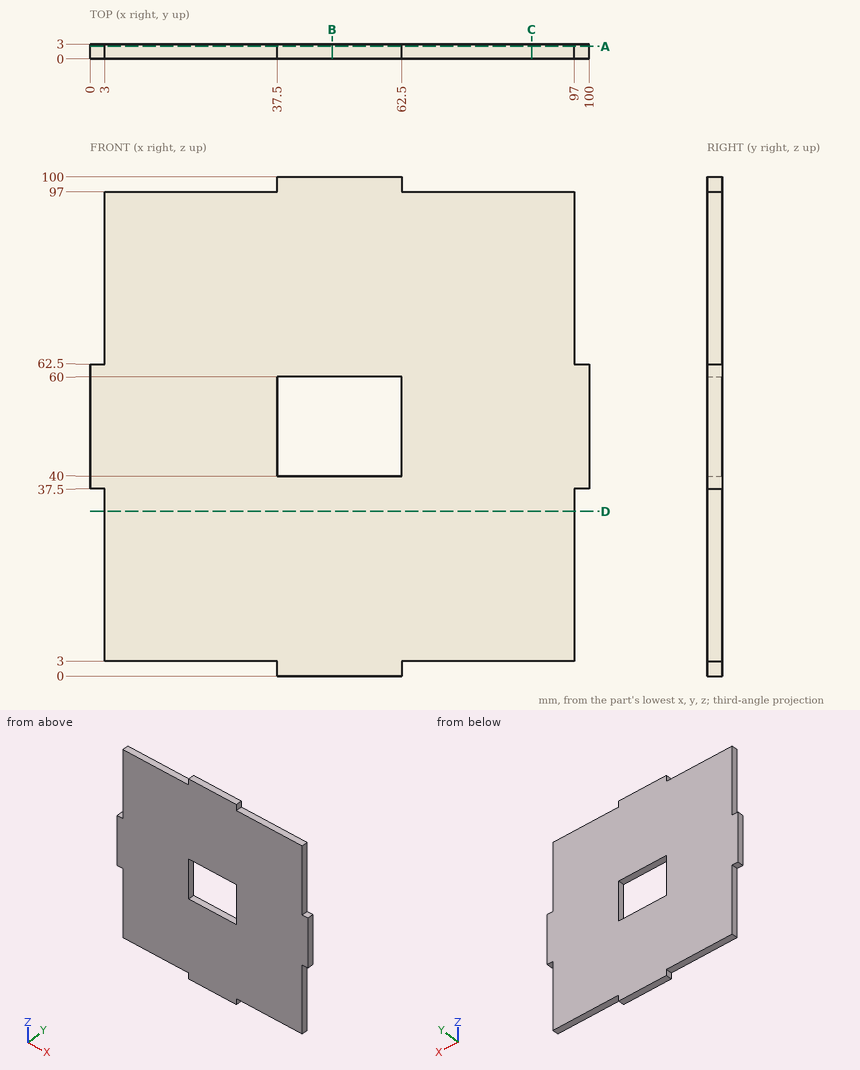
Could you check a few things on this drawing? It's one solid part, dimensions in mm from its lowest x, y, z. Coordinates: 2 decimals unless noted, no trailing zeros. Order: outer loops, then holes, each group sorted by start corner. A loop starts at its lowest first (then second) coordinate and runs counter-clockwise, first axis right, second up. Notation, with made-up numbers: (-21, 44.5) - (-14, 44.5) arc R10 ccw to (-14, 55.5) - close; hole circle Ø10 at (49, 81.5). An arc over 180 degrees is marked (long way). Answer as a JSON object with one key per item and string values. Group by question number.
Q1. Will these pins go through, and if not, where does the flat tip stop? P1, Ø0.9, axis at x = 2, y = 1, coming from the +Z side; P2, Ø1.5, axis at x = 80, y = 1.5, coming from the +Z side; P3, Ø1.5, axis at y = 1, z = 74.5, coming from the -X side; P4, Ø1.5, axis at y = 1.5, z = 55, coming from the -X side.
Q2. Imagine slicing it at D-D (z = 33). Please give me the cut outline in (x, y), and give its area (3 significant figures).
Q3. Imagine slicing it at C-C (x = 88.5). Please give me the cut outline in (y, z).
Q4. I need wall thicknesses on line 1 (X direction, y = 1.35, z = 50); line 2 (Z direction, x = 57, y = 0.9); line 3 (X direction, y = 1.75, z = 69). Which ranges of each line are inside material? Lowest first, please. Write a range as from..to.
Q5. Imagine slicing it at A-A (y = 2.5). Please give me the cut outline in (x, z), and give its area (3 significant figures).
Q6. Imagine slicing it at B-B (x = 48.5). Please give me the cut outline in (y, z), and give its area (3 significant figures).
Determined:
{
 "1": {"P1": "stops at z = 62.5", "P2": "stops at z = 97", "P3": "stops at x = 3", "P4": "stops at x = 0"},
 "2": {"outline": "(3, 0) - (97, 0) - (97, 3) - (3, 3) - close", "area": "282 mm2"},
 "3": {"outline": "(0, 3) - (3, 3) - (3, 97) - (0, 97) - close"},
 "4": {"line 1": "x = 0..37.5, 62.5..100", "line 2": "z = 0..40, 60..100", "line 3": "x = 3..97"},
 "5": {"outline": "(0, 37.5) - (3, 37.5) - (3, 3) - (37.5, 3) - (37.5, 0) - (62.5, 0) - (62.5, 3) - (97, 3) - (97, 37.5) - (100, 37.5) - (100, 62.5) - (97, 62.5) - (97, 97) - (62.5, 97) - (62.5, 100) - (37.5, 100) - (37.5, 97) - (3, 97) - (3, 62.5) - (0, 62.5) - close; hole (37.5, 40) - (62.5, 40) - (62.5, 60) - (37.5, 60) - close", "area": "8,640 mm2"},
 "6": {"outline": "(0, 0) - (3, 0) - (3, 40) - (0, 40) - close; (0, 60) - (3, 60) - (3, 100) - (0, 100) - close", "area": "240 mm2"}
}
